from build123d import *

# Parameters (mm, degrees)
SKETCH_1_R          = 2
EXTRUDE_1_DEPTH     = 0.8
SKETCH_2_R          = 1
EXTRUDE_2_DEPTH     = 5
FILLET_1_R          = 0.15
CHAMFER_1_SIZE      = 0.2
CUT_EXTRUDE_1_DEPTH = 0.5


with BuildPart() as part:
    # 草图1 → 凸台-拉伸1 (new body)
    with BuildSketch(Plane(origin=(0, 0, 0), x_dir=(1, 0, 0), z_dir=(0, 1, 0))):
        Circle(SKETCH_1_R)
    extrude(amount=EXTRUDE_1_DEPTH)

    # 草图2 → 凸台-拉伸2 (add)
    with BuildSketch(Plane.XZ):
        Circle(SKETCH_2_R)
    extrude(amount=EXTRUDE_2_DEPTH)

    # 圆角1
    fillet_1_edges = [part.edges().sort_by_distance(p)[0] for p in [
        (-2, 0, 0),
        (-2, 0.8, 0),
    ]]
    fillet(fillet_1_edges, radius=FILLET_1_R)

    # 倒角1
    chamfer_1_edges = [part.edges().sort_by_distance(p)[0] for p in [
        (-1, -5, 0),
    ]]
    chamfer(chamfer_1_edges, length=CHAMFER_1_SIZE)

    # 草图3 → 切除-拉伸1 (cut)
    with BuildSketch(Plane(origin=(0, 0.8, 0), x_dir=(1, 0, 0), z_dir=(0, 1, 0))):
        Polygon((0.75055535, 0), (0.375277675, 0.65), (-0.375277675, 0.65), (-0.75055535, 0), (-0.375277675, -0.65), (0.375277675, -0.65), align=None)
    extrude(amount=-CUT_EXTRUDE_1_DEPTH, mode=Mode.SUBTRACT)


solid = part.part
For this review, take the finished solid that the model builds, in its own axes (mm). A direction names the side the tool comes from. Round coordinates to 2 decimals unless told otherwise and drop trailing zeros. Order: outer loops, then holes, each group sorted by start corner. A loop starts at its lowest first (then second) coordinate and runs counter-clockwise, first axis right, second up. Notation, with made-up numbers: M 6.25,-5 L 58.25,-5 A21 cw 58.25,5 Z; hole C -6.75,-18 d4. An arc over 180 degrees is marked long. Use a Markdown table: item, result. Add a question column.
Item 1: Mouldability with a two-part tool opening along X and no side actions: class faces 3 (the cylindrical face through (0, -2, -1)), 4 (the flat face through (0, 0.3, 0)), 5 (the flat face through (0, -5, 0)) as released by +X, released by -X, zero draft, split by the parting line, or undercut.
Item 2: Tool access review of faces 1 (the flat face through (0, 0.8, 1)), 2 (the flat face through (1, 0, 1)): name each direction out of +Z, -Z, +X, -X, +Y, -Y from which nothing blocks a thin tool from reaching the whole face with its end or side.
Item 3: Add section B-B, the plane y = -2.85. Give the boundary of the cut face in (x, z), then the cut area to 3 significant figures.
Item 4: Add section A-A, the plane x = 0. Give the boundary of the cut face in (y, z).
Item 5: To check wall thickness, follow line 1 along Z through (x, y) = (0.05, -2.75); line 2 along Y through (x, z) = (-1.1, -1.4); line 3 along Z through (x, y) = (0.25, 0.4). State the ranges of each line that lie inside material, in increasing order.
Geometry results:
| question | item | result |
|---|---|---|
| 1 | face 3 | split by the parting line |
| 1 | face 4 | undercut |
| 1 | face 5 | zero draft |
| 2 | face 1 | +Z, -Z, +X, -X, +Y |
| 2 | face 2 | -Y |
| 3 | outline | C 0,0 d2 |
| 3 | area | 3.14 mm² |
| 4 | outline | M -5,-0.8 L -4.8,-1 L 0,-1 L 0,-1.85 A0.15 ccw 0.15,-2 L 0.65,-2 A0.15 ccw 0.8,-1.85 L 0.8,-0.65 L 0.3,-0.65 L 0.3,0.65 L 0.8,0.65 L 0.8,1.85 A0.15 ccw 0.65,2 L 0.15,2 A0.15 ccw 0,1.85 L 0,1 L -4.8,1 L -5,0.8 Z |
| 5 | line 1 | z = -1 to 1 |
| 5 | line 2 | y = 0 to 0.8 |
| 5 | line 3 | z = -1.98 to -0.65, 0.65 to 1.98 |
